```python
from build123d import *

# Parameters (mm, degrees)
F0_W     = 336.55
F0_H     = 127
F1_DEPTH = 19.05
F3_DEPTH = 336.551
F5_DEPTH = 127.0010001


with BuildPart() as f1:
    # F0 (on Front) → F1 (new body)
    with BuildSketch(Plane.XZ):
        Rectangle(F0_W, F0_H)
    extrude(amount=F1_DEPTH)

    # F2 (on face) → F3 (cut, through all)
    with BuildSketch(Plane.YZ.offset(168.275)):
        with BuildLine():
            add(Edge.make_bspline(
                [(0, 63.5), (-13.8609133718, 63.5), (-9.1129885479, 55.0204556119), (-15.256598862, 52.3182653746)],
                knots=[0, 0, 0, 0, 19.4568359991, 19.4568359991, 19.4568359991, 19.4568359991], degree=3))
            Line((0, 63.5), (-19.05, 63.5))
            Line((-19.05, 63.5), (-19.05, 51.528967917))
            add(Edge.make_bspline(
                [(-15.256598862, 52.3182653746), (-16.2172018341, 51.8957561593), (-17.4440793365, 51.6144907855), (-19.05, 51.528967917)],
                knots=[19.4568359991, 19.4568359991, 19.4568359991, 19.4568359991, 22.4990690726, 22.4990690726, 22.4990690726, 22.4990690726], degree=3))
        make_face()
        with BuildLine():
            ThreePointArc((-19.05, 46.505666794), (-18.0177487141, 49.976120455), (-15.256598862, 52.3182653746))
            add(Edge.make_bspline(
                [(-15.256598862, 52.3182653746), (-16.2172018341, 51.8957561593), (-17.4440793365, 51.6144907855), (-19.05, 51.528967917)],
                knots=[19.4568359991, 19.4568359991, 19.4568359991, 19.4568359991, 22.4990690726, 22.4990690726, 22.4990690726, 22.4990690726], degree=3))
            Line((-19.05, 51.528967917), (-19.05, 46.505666794))
        make_face()
    extrude(amount=-F3_DEPTH, mode=Mode.SUBTRACT)

    # F4 (on face) → F5 (cut, through all)
    with BuildSketch(Plane(origin=(0, 0, -63.5), x_dir=(1, 0, 0), z_dir=(0, 0, -1))):
        Polygon((-149.225, 0), (-168.275, 19.05), (-168.275, 0), align=None)
    extrude(amount=-F5_DEPTH, mode=Mode.SUBTRACT)


solid = f1.part
```
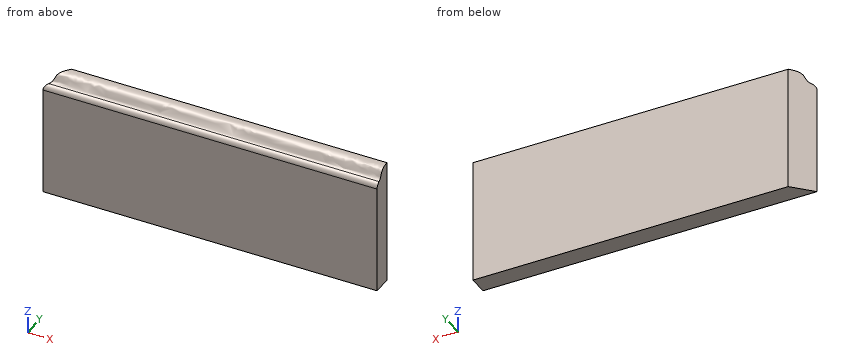
Design review of the part built by this model. Coordinates are the model's own, in mm. Round coordinates to 2 decimals unless told otherwise and drop trailing zeros. Write each loop counter-clockwise with the first axis right and the second up, starting at its lowest first coordinate (ties: lowest second). Pieces come first, ordered by that corner, then holes. Notation, with made-up numbers: (-4, 15) -> (26, 15) arc R19 cw to (26, 22) -> close; hole circle Ø5 at (53.5, -33). An arc over 180 degrees is marked (long way). Answer in a Markdown table with one row per item.
Q1. Take a section at A-A, the plane z = 41. State the section outline as (x, y) points (3 decimals), then the cut area to 3 significant figures.
The answers:
| item | result |
|---|---|
| outline | (-168.275, -19.05) -> (168.275, -19.05) -> (168.275, 0) -> (-149.225, 0) -> close |
| area | 6,230 mm² |
Q2. Clearance check with flat-ended pins moving along their axes: pin 1 Ø12 at (x, z) = (-93, 41) entering from +Y; pin 2 Ø3 at (x, y) = (-47, -11) entering from +Z. State where each tip first meets the part, or that it passes through.
The answers:
| item | result |
|---|---|
| pin 1 | y = 0 |
| pin 2 | z = 60.45 |
Q3. To check wall thickness, follow L1, parallel to Z at x = 26.5, y = -1; L2, parallel to Z at x = 96, y = -13.5; L3, parallel to X at y = -2.25, z = -34 (3 decimals). State the ranges of each line that lie inside material, in increasing order. Write a range as [from, to].
The answers:
| item | result |
|---|---|
| L1 | [-63.5, 63.48] |
| L2 | [-63.5, 53.48] |
| L3 | [-151.475, 168.275] |
